from build123d import *

# Parameters (mm, degrees)
SKETCH2_R           = 5.9
BOSS_EXTRUDE1_DEPTH = 8.6
SKETCH3_W           = 0.5
SKETCH3_H           = 2
BOSS_EXTRUDE2_DEPTH = 3.4


with BuildPart() as part:
    # Sketch1 → Revolve1 (revolve)
    with BuildSketch(Plane.XY, mode=Mode.PRIVATE) as revolve1_sk:
        with BuildLine():
            Line((0, 0), (-8.75, 0))
            Line((-8.75, 0), (-8.75, 1))
            Line((-8.75, 1), (-6.5, 5.1))
            Line((-6.5, 5.1), (-6.25, 5.1))
            Line((-6.25, 5.1), (-6.25, 5.35))
            ThreePointArc((-6.25, 5.35), (-3.273568389, 6.801180735), (0, 7.3))
            Line((0, 7.3), (0, 0))
        make_face()
    revolve(revolve1_sk.sketch.rotate(Axis((0, 7.3, 0), (0, -1, 0)), 270), axis=Axis((0, 7.3, 0), (0, -1, 0)))

    # Sketch2 → Boss-Extrude1 (add)
    with BuildSketch(Plane.XZ):
        with Locations(Location((0, 0, 0), (0, 0, 90))):
            Circle(SKETCH2_R)
    extrude(amount=BOSS_EXTRUDE1_DEPTH)

    # Sketch3 → Boss-Extrude2 (add)
    with BuildSketch(Plane.XZ.offset(8.6)):
        with Locations((-3.25, 0)):
            Rectangle(SKETCH3_W, SKETCH3_H)
        with Locations((3.25, 0)):
            Rectangle(SKETCH3_W, SKETCH3_H)
    extrude(amount=BOSS_EXTRUDE2_DEPTH)


solid = part.part
Read the model definition and answer for the solid it produces. Units are mm, in the model's axes. A direction names the side the tool comes from. Coordinates: 2 decimals unless noted, no trailing zeros. Write each loop counter-clockwise with the first axis right and the second up, starting at its lowest first coordinate (ties: lowest second). Pieces come first, ordered by that corner, then holes. Notation, with made-up numbers: (-11, 37) -> (43, 37) arc R19 ccw to (43, 49) -> close; hole circle Ø10 at (2.25, -7). An arc over 180 degrees is marked (long way). Return JSON: item names as keys, results as strings.
(1) The part is cut by section D-D on y = -3. Give the vertices of the cut face in (x, z).
Answers below:
{"outline": "circle Ø11.8 at (0, 0)"}
(2) For a pull along X with two mould halves and no side action, classify faces 4 (the cylindrical face through (5.324, 0.507, -6.944)), 5 (the flat face through (-3.5, -10, 0)), 6 (the flat face through (3, -10, 0)), 7 (the flat face through (-3, -10, 0)) as pulls with the +X half, pulls with the -X half, needs draft (parallel to the pull), parting line crosses it, or undercut.
Answers below:
{"face 4": "parting line crosses it", "face 5": "pulls with the -X half", "face 6": "undercut", "face 7": "undercut"}
(3) The part is cut by section C-C on z = 0. Give the vertices of the cut face in (x, y), then the cut area to 3 significant figures.
Answers below:
{"outline": "(-8.75, 0) -> (-5.9, 0) -> (-5.9, -8.6) -> (-3.5, -8.6) -> (-3.5, -12) -> (-3, -12) -> (-3, -8.6) -> (3, -8.6) -> (3, -12) -> (3.5, -12) -> (3.5, -8.6) -> (5.9, -8.6) -> (5.9, 0) -> (8.75, 0) -> (8.75, 1) -> (6.5, 5.1) -> (6.25, 5.1) -> (6.25, 5.35) arc R10.99 ccw to (-6.25, 5.35) -> (-6.25, 5.1) -> (-6.5, 5.1) -> (-8.75, 1) -> close", "area": "205 mm^2"}
(4) The part is cut by section B-B on x = 0. Give the vertices of the cut face in (y, z).
Answers below:
{"outline": "(-8.6, -5.9) -> (0, -5.9) -> (0, -8.75) -> (1, -8.75) -> (5.1, -6.5) -> (5.1, -6.25) -> (5.35, -6.25) arc R10.99 ccw to (5.35, 6.25) -> (5.1, 6.25) -> (5.1, 6.5) -> (1, 8.75) -> (0, 8.75) -> (0, 5.9) -> (-8.6, 5.9) -> close"}
(5) Consider line 1 along X through (y, z) = (-1.25, 0.25); line 2 along X through (y, z) = (3, 2.5); line 3 along Y through (x, z) = (-4.75, 0). Determine where each line is inside the solid, lowest interval first. Write a range as from..to.
Answers below:
{"line 1": "-5.89..5.89", "line 2": "-7.23..7.23", "line 3": "-8.6..6.22"}
(6) The part is cut by section A-A on y = -10. Give the vertices of the cut face in (x, z), then the cut area to 3 significant figures.
Answers below:
{"outline": "(-3.5, -1) -> (-3, -1) -> (-3, 1) -> (-3.5, 1) -> close; (3, -1) -> (3.5, -1) -> (3.5, 1) -> (3, 1) -> close", "area": "2.00 mm^2"}
(7) Which of the six approach directions +Z, -Z, +X, -X, +Y, -Y give full straight-line access (tool end or side, diameter ignored) to faces 1 (the flat face through (3.5, -10, 0)), 2 (the conical face through (6.452, 4.901, -1.433)), 3 (the cylindrical face through (5.76, -4.24, -1.28))?
Answers below:
{"face 1": "+Z, -Z, +X, -Y", "face 2": "+Y", "face 3": "-Y"}
(8) Each of these flat-tipped pins is pushed along its axis until it touches: P1, Ø1, axis at y = -10, z = 0, coming from the -X side; P2, Ø0.6, axis at x = 3, y = -11, coming from the -Z side; P3, Ø1, axis at y = -4, z = -5.5, coming from the +X side. Where does it stop, or does it pass through?
Answers below:
{"P1": "x = -3.5", "P2": "z = -1", "P3": "x = 3.13"}
